The model under review builds one solid part; all positions refer to its coordinate system, in mm. A direction names the side the tool comes from. Coordinates: 2 decimals unless noted, no trailing zeros. Order: outer loops, then holes, each group sorted by start corner. A loop starts at its lowest first (then second) coordinate and runs counter-clockwise, first axis right, second up. Notation, with made-up numbers: M 63,-0.5 L 107,-0.5 A25 cw 107,20.5 Z; hole C 36,39.5 d9. An arc over 180 degrees is marked long. Write each question's results on one line, items separated by ' | '.
from build123d import *

# Parameters (mm, degrees)
SKETCH1_W           = 34
SKETCH1_H           = 29
BOSS_EXTRUDE1_DEPTH = 2
SKETCH1_4_W         = 6.75
SKETCH1_4_H         = 26.25
BOSS_EXTRUDE2_DEPTH = 2.5
SKETCH2_W           = 34
SKETCH2_H           = 2.75
BOSS_EXTRUDE7_DEPTH = 2.5
CUT_EXTRUDE1_DEPTH  = 23.483327156
SKETCH4_R           = 1.75
CUT_EXTRUDE2_DEPTH  = 23.79254264
SKETCH5_W           = 16.5
SKETCH5_H           = 22.75
CUT_EXTRUDE3_DEPTH  = 1
FILLET1_SIZE        = 6
FILLET1_SIZE_2      = 3


with BuildPart() as part:
    # Sketch1 → Boss-Extrude1 (new body)
    with BuildSketch(Plane(origin=(0, 0, 0), x_dir=(1, 0, 0), z_dir=(0, 1, 0))):
        Rectangle(SKETCH1_W, SKETCH1_H)
    extrude(amount=BOSS_EXTRUDE1_DEPTH)

    # Sketch1<4> → Boss-Extrude2 (add)
    with BuildSketch(Plane(origin=(0, 0, 0), x_dir=(1, 0, 0), z_dir=(0, 1, 0))):
        with Locations((-13.625, -1.375)):
            Rectangle(SKETCH1_4_W, SKETCH1_4_H)
        with Locations((13.625, -1.375)):
            Rectangle(SKETCH1_4_W, SKETCH1_4_H)
    extrude(amount=-BOSS_EXTRUDE2_DEPTH)

    # Sketch2 → Boss-Extrude7 (add)
    with BuildSketch(Plane.XZ):
        with Locations((0, -13.125)):
            Rectangle(SKETCH2_W, SKETCH2_H)
    extrude(amount=BOSS_EXTRUDE7_DEPTH)

    # Sketch3 → Cut-Extrude1 (cut, through all)
    with BuildSketch(Plane.XZ):
        Polygon((-8.25, 12.5), (-8.25, 8.697540798), (8.25, -0.828738644), (8.25, 12.5), align=None)
        Polygon((-8.25, 4.078738644), (-8.25, -10.25), (8.25, -10.25), (8.25, -5.447540798), align=None)
    extrude(amount=-CUT_EXTRUDE1_DEPTH, mode=Mode.SUBTRACT)

    # Sketch4 → Cut-Extrude2 (cut, through all)
    with BuildSketch(Plane.XZ.offset(2.5)):
        with Locations(Location((14, 6.5, 0), (0, 0, 270))):
            Circle(SKETCH4_R)
        with Locations(Location((-14, 6.5, 0), (0, 0, 270))):
            Circle(SKETCH4_R)
    extrude(amount=-CUT_EXTRUDE2_DEPTH, mode=Mode.SUBTRACT)

    # Sketch5 → Cut-Extrude3 (cut)
    with BuildSketch(Plane.XZ):
        with Locations((0, 1.125)):
            Rectangle(SKETCH5_W, SKETCH5_H)
    extrude(amount=-CUT_EXTRUDE3_DEPTH, mode=Mode.SUBTRACT)

    # Fillet1
    # an asymmetric fillet: 6, 3 mm, written as the material it takes off along each edge
    with BuildSketch(Plane(origin=(-17, 17, 14.5), x_dir=(1, 0, 0), z_dir=(0, -1, 0)), Plane(origin=(17, -17.5, 14.5), x_dir=(-1, 0, 0), z_dir=(0, 1, 0))) as fillet1_piece_1:
        with BuildLine():
            Bezier((FILLET1_SIZE, 0), (0, 0), (0, -FILLET1_SIZE_2), weights=[1, 0.707106781, 1])
            Line((0, -FILLET1_SIZE_2), (0, 0))
            Line((0, 0), (FILLET1_SIZE, 0))
        make_face()
    extrude(amount=34.5, mode=Mode.SUBTRACT)
    with BuildSketch(Plane(origin=(-17, 17, -14.5), x_dir=(1, 0, 0), z_dir=(0, -1, 0)), Plane(origin=(17, -17.5, -14.5), x_dir=(-1, 0, 0), z_dir=(0, 1, 0))) as fillet1_piece_2:
        with BuildLine():
            Bezier((FILLET1_SIZE, 0), (0, 0), (0, FILLET1_SIZE_2), weights=[1, 0.707106781, 1])
            Line((0, FILLET1_SIZE_2), (0, 0))
            Line((0, 0), (FILLET1_SIZE, 0))
        make_face()
    extrude(amount=34.5, mode=Mode.SUBTRACT)


solid = part.part
1) To check wall thickness, follow line 1 along X through (y, z) = (0.2, 6.5); line 2 along X through (y, z) = (-0.4, 6.5); line 3 along X through (y, z) = (-1.2, 4). State the ranges of each line that lie inside material, in increasing order.
Solutions:
line 1: -17 to -15.75, -12.25 to -8.25, 8.25 to 12.25, 15.75 to 17 | line 2: -17 to -15.75, -12.25 to -10.25, 10.25 to 12.25, 15.75 to 17 | line 3: -17 to -10.25, 10.25 to 17
2) For pin 1 (4 mm diameter, centred on x = -8, z = 9.5, fed in from -Y), flat-tipped, find the tip position at first contact; note if it passes through.
Solutions:
pin 1: y = 0
3) Take a section at A-A on z = -8. State the section outline as (x, y) points, plus the area to 4 significant figures.
Solutions:
outline: M -17,-2.5 L -10.25,-2.5 L -10.25,0 L -8.25,0 L -8.25,2 L -17,2 Z; M 8.25,0 L 10.25,0 L 10.25,-2.5 L 17,-2.5 L 17,2 L 8.25,2 Z | area: 68.75 mm2
4) Take a section at B-B on x = -7.5. State the section outline as (y, z) points.
Solutions:
outline: M -2.5,-14.5 L 2,-14.5 L 2,-10.25 L 0,-10.25 L 0,-11.75 L -2.5,-11.75 Z; M 0,12.5 L 2,12.5 L 2,14.5 L 0,14.5 Z; M 1,3.65 L 2,3.65 L 2,8.26 L 1,8.26 Z
5) For faces 1 (the flat face through (0, 2, 0)), 2 (the flat face through (0, 1, 12.5)), 3 (the flat face through (8.25, 1, 1)), 4 (the flat face through (0, -1, -11.75)), list the 3-axis set-ups (+Z, -Z, +X, -X, +Y, -Y) from which the entire face can be reached by the end or side of a thin tool; tool diameter is ignored.
Solutions:
face 1: +Z, -Z, +X, -X, +Y | face 2: +Y, -Y | face 3: -Y | face 4: +Z, -Y
6) Take a section at C-C on z = 6.5. State the section outline as (x, y) points.
Solutions:
outline: M -17,-2.5 L -15.75,-2.5 L -15.75,2 L -17,2 Z; M -12.25,-2.5 L -10.25,-2.5 L -10.25,0 L -8.25,0 L -8.25,1 L -4.44,1 L -4.44,2 L -12.25,2 Z; M 8.25,0 L 10.25,0 L 10.25,-2.5 L 12.25,-2.5 L 12.25,2 L 8.25,2 Z; M 15.75,-2.5 L 17,-2.5 L 17,2 L 15.75,2 Z
7) Take a section at D-D on z = 0. State the section outline as (x, y) points.
Solutions:
outline: M -17,-2.5 L -10.25,-2.5 L -10.25,0 L -8.25,0 L -8.25,2 L -17,2 Z; M -1.19,1 L 6.81,1 L 6.81,2 L -1.19,2 Z; M 8.25,0 L 10.25,0 L 10.25,-2.5 L 17,-2.5 L 17,2 L 8.25,2 Z
8) The part is to be moulded in two halves that separate along X. For faces 5 (the flat face through (17, 0, 0)), 6 (the flat face through (-8.25, 1, 1)), 7 (the flat face through (0, 0, -14.5)), say which applies: pulls with the +X half, pulls with the -X half, needs draft (parallel to the pull), parting line crosses it, or undercut.
Solutions:
face 5: pulls with the +X half | face 6: undercut | face 7: needs draft
